Geometry check sheet. Reference: the model listing, model coordinates, mm. Give positions to 0.01 mm unless a question says otherwise; leave off trailing zeros. Loops run counter-clockwise (first coordinate to the right, second up) from the corner with the lowest first, then second, coordinate; pieces in that order, holes last. Notation, with made-up numbers: (87, 56.5) -> (130, 56.5) arc R30 cw to (130, 91.5) -> close; hole circle Ø11 at (-35.5, -27). An arc over 180 degrees is marked (long way). One line per item, written item: value. Start each with the question number.
(1) Sectioned sample at A-A, the plane z = 2.85. Record the cut outline in (x, y).
(2) Sectioned sample at D-D, the plane x = 16.5. Record the cut outline in (y, z), then the cut area to 3 significant figures.
(3) Scan lines: line 1 along Y through (x, z) = (35, 2.05); line 2 along X through (y, z) = (0, 0.8); line 3 along Y through (x, z) = (0, 3). Record each from-to range of solid material in increasing order. Write a range as from..to.
(4) Gauge pin test, flat ends, axial feed: pin 1 Ø1 at (x, y) = (19, 11.5) entering from +Z; pin 2 Ø1.5 at (x, z) = (13.5, 1.5) entering from +Y. Record the tip position at first contact, or that the pin passes through.
(5) Sectioned sample at B-B, the plane x = 35. Record the cut outline in (y, z).
(6) Sectioned sample at C-C, the plane y = 1.5. Record the cut outline in (x, z).
Autodesk Inventor part; units mm, degrees
ref_plane "YZ Plane" through (0, 0, 0) normal (1, 0, 0) x (0, 1, 0)
ref_plane "XZ Plane" through (0, 0, 0) normal (0, 1, 0) x (-1, 0, 0)
ref_plane "XY Plane" through (0, 0, 0) normal (0, 0, 1) x (1, 0, 0)
sketch "スケッチ1" plane through (0, 0, 0) normal (0, 0, 1) x (1, 0, 0)
  line L0 (0, 0) -> (35, 11.927) construction
  line L1 (33.7098, 15.7132) -> (-1.2902, 3.7862)
  line L2 (-4, 0) -> (-4, -12.5)
  line L3 (-4, -12.5) -> (39, -12.5)
  line L4 (39, -12.5) -> (39, 11.927)
  arc A0 (-1.2902, 3.7862) -> (-4, 0) centre (0, 0) ccw
  arc A1 (39, 11.927) -> (33.7098, 15.7132) centre (35, 11.927) ccw
  dimension "d0" = 35
  dimension "d1" = 11.927
  dimension "d2" = 4
  dimension "d12" = 12.5
extrude "押し出し1" add sketch "スケッチ1" along normal blind 5
hole "穴1" at (0, 0, 0) at (35, 11.927, 0) direction (0, 0, 1) diameter 4 end through all
properties part number "COXA_ROLL_COUPLER_BACK"
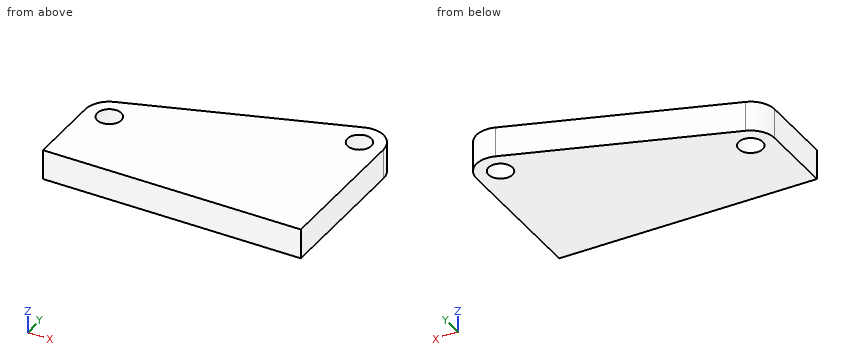
Calculated:
1. outline: (-4, -12.5) -> (39, -12.5) -> (39, 11.93) arc R4 ccw to (33.71, 15.71) -> (-1.29, 3.79) arc R4 ccw to (-4, 0) -> close; hole circle Ø4 at (0, 0); hole circle Ø4 at (35, 11.93)
2. outline: (-12.5, 0) -> (9.85, 0) -> (9.85, 5) -> (-12.5, 5) -> close
2. area: 112 mm2
3. line 1: y = -12.5..9.93, 13.93..15.93
3. line 2: x = -4..-2, 2..39
3. line 3: y = -12.5..-2, 2..4.23
4. pin 1: passes through
4. pin 2: stops at y = 9.08
5. outline: (-12.5, 0) -> (9.93, 0) -> (9.93, 5) -> (-12.5, 5) -> close; (13.93, 0) -> (15.93, 0) -> (15.93, 5) -> (13.93, 5) -> close
6. outline: (-3.71, 0) -> (-1.32, 0) -> (-1.32, 5) -> (-3.71, 5) -> close; (1.32, 0) -> (39, 0) -> (39, 5) -> (1.32, 5) -> close
